Geometry: see drawing. Coordinates: mm, zero at the bounding-box minimum. Round coordinates to 2 decimals unless told otherwise and drop trailing zeros. Loops run counter-clockwise (first coordinate to the right, second up) from the corner with the lowest first, then second, coordinate; pieces in that order, holes last. Notation, with made-up numbers: (-22.75, -18.75) -> (35.25, -18.75) arc R24 cw to (35.25, -1.75) -> close; hole circle Ø8 at (2.5, 49.25). An arc over 180 degrees is marked (long way). Answer in a Markdown table with one row per item.
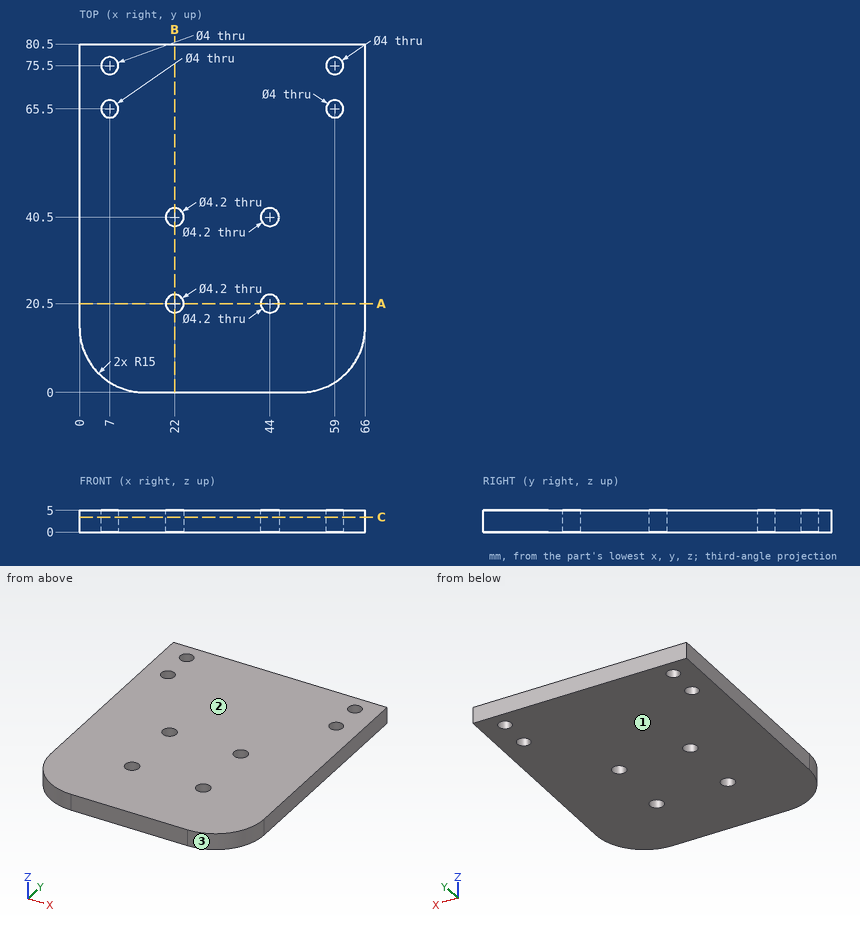
Item 1: Section query C-C, the plane z = 3.45. State how many separate pieces and enclosed holes the cut face has, and give its area (3 significant figures).
Ans:
| item | result |
|---|---|
| separate pieces | 1 |
| enclosed holes | 8 |
| area | 5,110 mm2 |
Item 2: Mould query, pull axis Z, two halves, no side actions, for the marked faces 1, 2 and 3. Classes: released by +Z, released by -Z, zero draft, split by the parting line, or undercut.
Ans:
| item | result |
|---|---|
| face 1 | released by -Z |
| face 2 | released by +Z |
| face 3 | zero draft |
Item 3: Section query B-B, the plane x = 22. Output: boundary loops of the cut face in (y, z).
Ans:
| item | result |
|---|---|
| outline | (0, 0) -> (18.4, 0) -> (18.4, 5) -> (0, 5) -> close; (22.6, 0) -> (38.4, 0) -> (38.4, 5) -> (22.6, 5) -> close; (42.6, 0) -> (80.5, 0) -> (80.5, 5) -> (42.6, 5) -> close |
Item 4: Ray query, L1, parallel to X at y = 65.5, z = 2.2; L2, parallel to Y at x = 22, z = 3.9; L3, parallel to Y at x = 7, z = 1.6. Return the intervals inside material, ascending.
Ans:
| item | result |
|---|---|
| L1 | 0 to 5, 9 to 57, 61 to 66 |
| L2 | 0 to 18.4, 22.6 to 38.4, 42.6 to 80.5 |
| L3 | 2.31 to 63.5, 67.5 to 73.5, 77.5 to 80.5 |
Item 5: Section query A-A, the plane y = 20.5. Output: boundary loops of the cut face in (x, z).
Ans:
| item | result |
|---|---|
| outline | (0, 0) -> (19.9, 0) -> (19.9, 5) -> (0, 5) -> close; (24.1, 0) -> (41.9, 0) -> (41.9, 5) -> (24.1, 5) -> close; (46.1, 0) -> (66, 0) -> (66, 5) -> (46.1, 5) -> close |
